```python
from build123d import *

# Parameters (mm, degrees)
F0_W     = 25
F0_H     = 19
F1_DEPTH = 20
F3_T     = -0.2
F2_R     = 2.75
F4_DEPTH = 25
F5_W     = 20
F5_H     = 1.2
F6_DEPTH = 1
F7_W     = 5
F7_H     = 4.8
F8_DEPTH = 24.9


with BuildPart() as f1:
    # F0 (on Front) → F1 (new body)
    with BuildSketch(Plane.XZ):
        with Locations((-12.5, 9.5)):
            Rectangle(F0_W, F0_H)
    extrude(amount=F1_DEPTH)

    # F3 (hollow: no face is removed)
    offset(amount=F3_T, mode=Mode.SUBTRACT)

    # F2 (on Front) → F4 (cut)
    with BuildSketch(Plane.XZ):
        with Locations((-12.5, 13)):
            Circle(F2_R)
    extrude(amount=F4_DEPTH, mode=Mode.SUBTRACT)

    # F5 (on face) → F6 (cut)
    with BuildSketch(Plane.XY.offset(19)):
        with Locations((-12.5, -10)):
            Rectangle(F5_W, F5_H)
    extrude(amount=-F6_DEPTH, mode=Mode.SUBTRACT)

    # F7 (on face) → F8 (cut)
    with BuildSketch(Plane.YZ):
        with Locations((-10, 2.5)):
            Rectangle(F7_W, F7_H)
    extrude(amount=-F8_DEPTH, mode=Mode.SUBTRACT)


solid = f1.part
```
Work out the finished part from the listing and answer in its coordinate system (mm). A direction names the side the tool comes from. Coordinates: 2 decimals unless noted, no trailing zeros. Order: outer loops, then holes, each group sorted by start corner. A loop starts at its lowest first (then second) coordinate and runs counter-clockwise, first axis right, second up. Notation, with made-up numbers: (45, 84.25) - (56, 84.25) arc R20 cw to (56, 96.25) - close; hole circle Ø10 at (9.25, 13). An arc over 180 degrees is marked (long way). Answer as a JSON object with one key per item and string values.
1. Find section D-D on y = -14. Determine the outline of the cut face in (x, z), plus the area to 3 significant figures.
Output values:
{"outline": "(-25, 0) - (0, 0) - (0, 19) - (-25, 19) - close; hole (-24.8, 0.2) - (-0.2, 0.2) - (-0.2, 18.8) - (-24.8, 18.8) - close", "area": "17.4 mm²"}
2. The mould has two halves that part along Z. Classify faces 1 (the face through (-13, -0.2, 10)), 2 (the face through (-13, -8, 19)), 3 (the face through (-25, -10, 9)): +Z half, -Z half, draft (parallel to the pull), parting line (faces both ways), or undercut.
Output values:
{"face 1": "undercut", "face 2": "+Z half", "face 3": "draft"}
3. Find section C-C on x = -12.5. Determine the outline of the cut face in (y, z).
Output values:
{"outline": "(-20, 0) - (0, 0) - (0, 10.25) - (-0.2, 10.25) - (-0.2, 0.2) - (-7.5, 0.2) - (-7.5, 0.1) - (-12.5, 0.1) - (-12.5, 0.2) - (-19.8, 0.2) - (-19.8, 10.25) - (-20, 10.25) - close; (-20, 15.75) - (-19.8, 15.75) - (-19.8, 18.8) - (-10.6, 18.8) - (-10.6, 19) - (-20, 19) - close; (-9.4, 18.8) - (-0.2, 18.8) - (-0.2, 15.75) - (0, 15.75) - (0, 19) - (-9.4, 19) - close"}
4. Consider line 1 (X direction, y = -18.25, z = 1); line 2 (Y direction, x = -19, z = 12); line 3 (Z direction, x = -12.5, y = -19.9). Determine where each line is inside the solid, lowest interval first.
Output values:
{"line 1": "x = -25 to -24.8, -0.2 to 0", "line 2": "y = -20 to -19.8, -0.2 to 0", "line 3": "z = 0 to 10.25, 15.75 to 19"}
5. This flat-tipped pin is pushed along its axis until it touches: P1, Ø4.5, axis at x = -12.5, z = 13, coming from the -Y side. Where does it stop, or does it pass through?
Output values:
{"P1": "passes through"}
6. Find section B-B on z = 13. Determine the outline of the cut face in (x, y), plus the area to 3 significant figures.
Output values:
{"outline": "(-25, -20) - (-15.25, -20) - (-15.25, -19.8) - (-24.8, -19.8) - (-24.8, -0.2) - (-15.25, -0.2) - (-15.25, 0) - (-25, 0) - close; (-9.75, -20) - (0, -20) - (0, 0) - (-9.75, 0) - (-9.75, -0.2) - (-0.2, -0.2) - (-0.2, -19.8) - (-9.75, -19.8) - close", "area": "15.6 mm²"}
7. Find section A-A on y = -10. Determine the outline of the cut face in (x, z).
Output values:
{"outline": "(-25, 0) - (0, 0) - (0, 0.1) - (-24.9, 0.1) - (-24.9, 4.9) - (-24.8, 4.9) - (-24.8, 18.8) - (-22.5, 18.8) - (-22.5, 19) - (-25, 19) - close; (-2.5, 18.8) - (-0.2, 18.8) - (-0.2, 4.9) - (0, 4.9) - (0, 19) - (-2.5, 19) - close"}
8. A tool of negligible diameter and unlimited length cuts with its end or side. For faces 4 (the face through (0, -10, 9)), 5 (the face through (-13, -12, 18.8)), from which of +Z, -Z, +X, -X, +Y, -Y can it reach the whole face along a straight path? Write none if from no direction.
Output values:
{"face 4": "+Z, -Z, +X, +Y, -Y", "face 5": "none"}
